Model file for the job. Use its own axes, mm. Coordinates: 2 decimals unless noted, no trailing zeros. Loops run counter-clockwise (first coordinate to the right, second up) from the corner with the lowest first, then second, coordinate; pieces in that order, holes last. Notation, with made-up numbers: (16.25, -10) -> (50.25, -10) arc R17 ccw to (50.25, 16) -> close; hole circle Ø6 at (33, 32.25). An arc over 180 degrees is marked (long way). Use one line per item in the form item = value.
Autodesk Inventor part; units mm, degrees
ref_plane "YZ Plane" through (0, 0, 0) normal (1, 0, 0) x (0, 1, 0)
ref_plane "XZ Plane" through (0, 0, 0) normal (0, 1, 0) x (-1, 0, 0)
ref_plane "XY Plane" through (0, 0, 0) normal (0, 0, 1) x (1, 0, 0)
sketch "Sketch1" plane through (0, 0, 0) normal (0, 0, 1) x (1, 0, 0)
  line L0 (-13, 12) -> (13, 12)
  line L1 (13, 12) -> (13, -12)
  line L2 (13, -12) -> (-13, -12)
  line L3 (-13, -12) -> (-13, 12)
  line L4 (-13, 3.25) -> (-15, 3.25)
  line L5 (-15, 3.25) -> (-15, -3.25)
  line L6 (-15, -3.25) -> (-13, -3.25)
  line L7 (-13, -3.25) -> (-13, 3.25)
  line L8 (13, 3.25) -> (15, 3.25)
  line L9 (15, 3.25) -> (15, -3.25)
  line L10 (15, -3.25) -> (13, -3.25)
  line L11 (13, -3.25) -> (13, 3.25)
  line L12 (-25.4, 25.4) -> (25.4, 25.4)
  line L13 (25.4, 25.4) -> (25.4, -25.4)
  line L14 (25.4, -25.4) -> (-25.4, -25.4)
  line L15 (-25.4, -25.4) -> (-25.4, 25.4)
  arc A0 (6.3617, 3.25) -> (-6.3617, 3.25) centre (0, 0) ccw
  circle A1 centre (-3, 12) radius 1.5
  line L16 (-13, 8) -> (-9, 12)
  line L17 (9, 12) -> (13, 8)
  line L18 (13, -8) -> (9, -12)
  line L19 (-13, -8) -> (-9, -12)
  line L20 (-14, 3.25) -> (14, 3.25)
  line L21 (-14, -3.25) -> (-6.3617, -3.25)
  arc A2 (6.3617, -3.25) -> (6.3617, 3.25) centre (0, 0) ccw
  arc A3 (-6.3617, 3.25) -> (-6.3617, -3.25) centre (0, 0) ccw
  arc A4 (-6.3617, -3.25) -> (6.3617, -3.25) centre (0, 0) ccw
  line L22 (-6.3617, -3.25) -> (14, -3.25)
  line L23 (-15, 3.25) -> (15, 3.25)
  line L24 (15, 3.25) -> (15, -3.25)
  line L25 (15, -3.25) -> (-15, -3.25)
  line L26 (-15, -3.25) -> (-15, 3.25)
  point P0 (-20.32, 20.32)
  point P1 (20.32, 20.32)
  point P2 (20.32, -20.32)
  point P3 (-20.32, -20.32)
  point P4 (-12, 0)
  point P5 (12, 0)
  dimension "d53" = 3.302
  dimension "d0" = 24
  dimension "d1" = 12
  dimension "d2" = 26
  dimension "d3" = 13
  dimension "d4" = 2
  dimension "d5" = 6.5
  dimension "d6" = 3.25
  dimension "d7" = 2
  dimension "d8" = 14.2875
  dimension "d9" = 50.8
  dimension "d10" = 25.4
  dimension "d11" = 50.8
  dimension "d12" = 25.4
  dimension "d13" = 3
  dimension "d14" = 10
  dimension "d15" = 4
  dimension "d16" = 4
  dimension "d17" = 4
  dimension "d18" = 4
  dimension "d19" = 4
  dimension "d20" = 5.08
  dimension "d21" = 5.08
  dimension "d22" = 5.08
  dimension "d23" = 5.08
  dimension "d34" = 40.64
  dimension "d35" = 40.64
  dimension "d61" = 12
  dimension "d62" = 12
extrude "Extrusion1" add sketch "Sketch1" against normal blind 3.175 contours L0 L16 L3 | L0 A1 L17 L1 L20 A0 L3 L16 | A1 L0 | L0 A1 | L20 A3 L21 L3 | L3 L6 L5 L4 | L21 A4 L22 L1 L18 L2 L19 L3 | A0 L20 | L20 A2 L22 A3 | L0 L1 L17 | L19 L2 L3 | L22 A4 | L20 L1 L22 A2 | L8 L9 L10 L1 | L18 L1 L2 | L12 L13 L14 L15
fillet "Fillet2" radius 4.7625 4 edges at (25.4, 25.4, -1.5875) (25.4, -25.4, -1.5875) (-25.4, 25.4, -1.5875) (-25.4, -25.4, -1.5875)
hole "Hole2" at (-20.32, 20.32, 0) at (20.32, 20.32, 0) at (20.32, -20.32, 0) at (-20.32, -20.32, 0) direction (0, 0, -1) diameter 3.302 end through all
extrude "Extrusion6" cut sketch "Sketch1" against normal through all contours A0 L20 | L20 A2 L22 A3 | L22 A4
hole "Hole3" at (-12, 0, 0) at (12, 0, 0) direction (0, 0, -1) diameter 3.3274 end through all
equation "\"d7\" = d4"
equation "\"d16\" = d15"
equation "\"d17\" = d15"
equation "\"d18\" = d15"
equation "\"d19\" = d15"
properties part number "BD gearbox mount top plate"
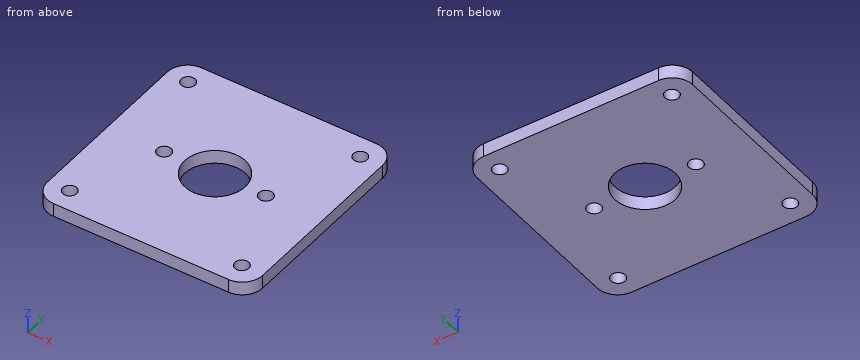
Q1. Band-saw the part on D-D, the plane z = -2.05. State how many separate pieces and enclosed holes the cut face has, and give its area (3 significant figures).
Result:
separate_pieces = 1
enclosed_holes = 7
area = 2,350 mm2
Q2. Band-saw the part on C-C, the plane x = 0. Write the cut outline in (y, z) (3 decimals).
Result:
outline = (-25.4, -3.175) -> (-7.144, -3.175) -> (-7.144, 0) -> (-25.4, 0) -> close; (7.144, -3.175) -> (25.4, -3.175) -> (25.4, 0) -> (7.144, 0) -> close
Q3. Band-saw the part on B-B, the plane x = 12. Write the cut outline in (y, z) (3 decimals).
Result:
outline = (-25.4, -3.175) -> (-1.664, -3.175) -> (-1.664, 0) -> (-25.4, 0) -> close; (1.664, -3.175) -> (25.4, -3.175) -> (25.4, 0) -> (1.664, 0) -> close
Q4. Wall check: line 1 along X through (y, z) = (0, -2.5); line 2 along X through (y, z) = (20.32, -1.85). Give the ranges that are in metal, low to high.
Result:
line_1 = -25.4 to -13.66, -10.34 to -7.14, 7.14 to 10.34, 13.66 to 25.4
line_2 = -25.4 to -21.97, -18.67 to 18.67, 21.97 to 25.4
Q5. Band-saw the part on A-A, the plane y = 0. Write the cut outline in (x, z) (3 decimals).
Result:
outline = (-25.4, -3.175) -> (-13.664, -3.175) -> (-13.664, 0) -> (-25.4, 0) -> close; (-10.336, -3.175) -> (-7.144, -3.175) -> (-7.144, 0) -> (-10.336, 0) -> close; (7.144, -3.175) -> (10.336, -3.175) -> (10.336, 0) -> (7.144, 0) -> close; (13.664, -3.175) -> (25.4, -3.175) -> (25.4, 0) -> (13.664, 0) -> close
